Geometry check sheet. Reference: drawing and pictorial views, mm from the part's lowest x, y, z. A direction names the side the tool comes from. Coordinates: 2 decimals unless noted, no trailing zeros. Loops run counter-clockwise (first coordinate to the right, second up) from the corner with the lowest first, then second, coordinate; pieces in that order, holes last. Notation, with made-up numbers: (-13, -37) -> (4, -37) arc R25 cw to (4, -16) -> close; hole circle Ø5 at (-14.5, 39.25). An arc over 180 degrees is marked (long way). Use CSV: the item, a comma, the result in double quotes.
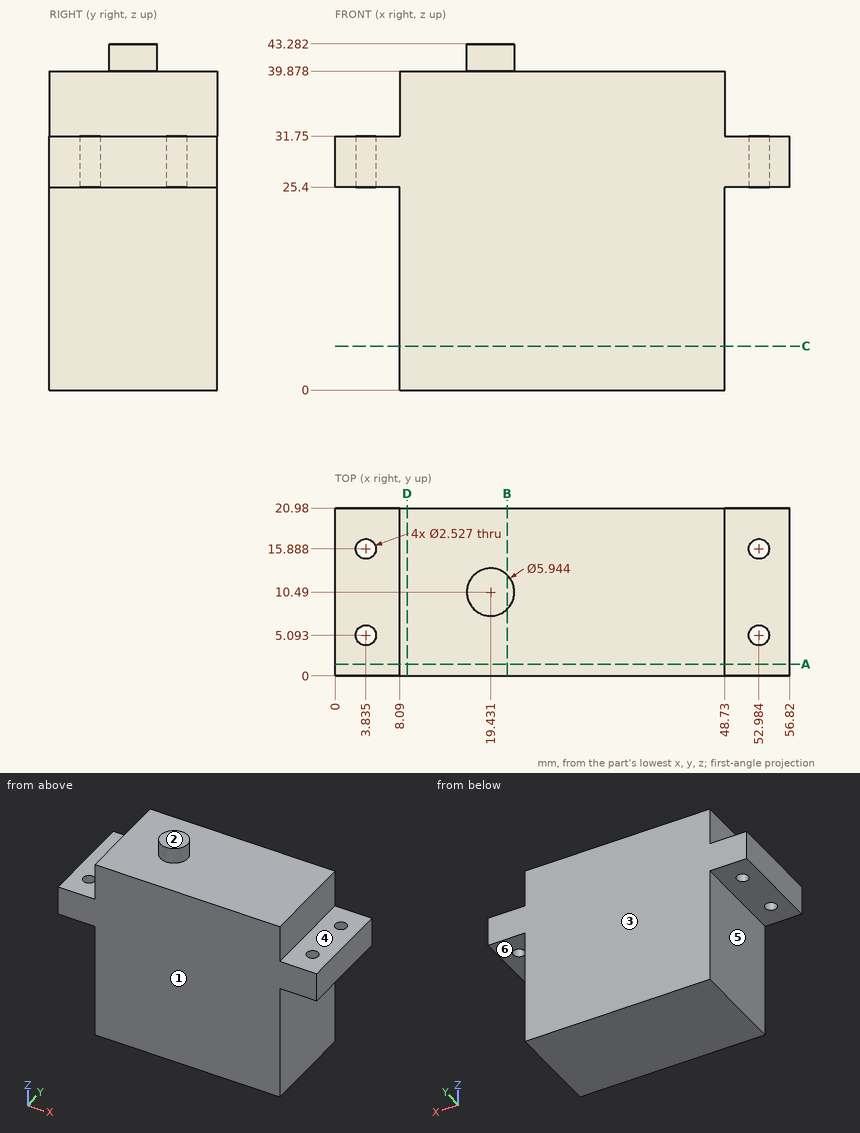
1) Access from +Z, -Z, +X, -X, +Y, -Y to the whole of each face (thin tool, end or side, straight path). Record for the marked faces 4, 5 and 6.
Answer below:
face 4,"+Z, +X, +Y, -Y"
face 5,"-Z, -X, +Y, -Y"
face 6,"-Z, +X, +Y, -Y"
2) Cross-section at C-C on z = 5.5. Record the boundary of the cut face in (x, y), and give its area (3 significant figures).
Answer below:
outline,"(8.09, 0) -> (48.73, 0) -> (48.73, 20.98) -> (8.09, 20.98) -> close"
area,"853 mm²"
3) Thickness scan on line 1 along X through (y, z) = (10.75, 38.5); line 2 along Z through (x, y) = (43.5, 14); line 3 along X through (y, z) = (10.75, 41.5). Record the ranges inside material, lowest first. Write a range as from..to.
Answer below:
line 1,"x = 8.09..48.73"
line 2,"z = 0..39.88"
line 3,"x = 16.47..22.39"
4) Cross-section at B-B on x = 21.5. Record the boundary of the cut face in (y, z).
Answer below:
outline,"(0, 0) -> (20.98, 0) -> (20.98, 39.88) -> (12.62, 39.88) -> (12.62, 43.28) -> (8.36, 43.28) -> (8.36, 39.88) -> (0, 39.88) -> close"
5) Cross-section at D-D on x = 9. Record the boundary of the cut face in (y, z).
Answer below:
outline,"(0, 0) -> (20.98, 0) -> (20.98, 39.88) -> (0, 39.88) -> close"
6) Go/stop test with flat-tipped pins: pin 1 Ø6.5 at (y, z) = (8.5, 17) entering from -X; pin 2 Ø1 at (x, y) = (24.5, 8) entering from -Z; pin 3 Ø3 at (x, y) = (3.84, 5.09) entering from +Z; pin 4 Ø9 at (x, y) = (4.5, 6.5) entering from +Z. Record where each tip stops, or that it passes through.
Answer below:
pin 1,"stops at x = 8.09"
pin 2,"stops at z = 0"
pin 3,"stops at z = 31.75"
pin 4,"stops at z = 39.88"
7) Cross-section at A-A on y = 1.5. Record the boundary of the cut face in (x, z), and give its area (3 significant figures).
Answer below:
outline,"(0, 25.4) -> (8.09, 25.4) -> (8.09, 0) -> (48.73, 0) -> (48.73, 25.4) -> (56.82, 25.4) -> (56.82, 31.75) -> (48.73, 31.75) -> (48.73, 39.88) -> (8.09, 39.88) -> (8.09, 31.75) -> (0, 31.75) -> close"
area,"1,720 mm²"
8) Draft check along Y on the marked faces 1, 2 and 3. Enter one of: released by +Y, released by -Y, zero draft, split by the parting line, or undercut.
Answer below:
face 1,"released by -Y"
face 2,"zero draft"
face 3,"released by +Y"
